from build123d import *

# Parameters (mm, degrees)
SKETCH1_R             = 22.5
SKETCH1_R_2           = 16.9
BOSS_EXTRUDE1_DEPTH   = 19
BOSS_EXTRUDE1_2_DEPTH = 19
BOSS_EXTRUDE2_DEPTH   = 9
CUT_EXTRUDE1_DEPTH    = 4
FILLET1_R             = 1
FILLET2_R             = 40
FILLET3_R             = 22.5
BOSS_EXTRUDE5_DEPTH   = 30
SKETCH6_R             = 27
CUT_EXTRUDE2_DEPTH    = 37
SKETCH7_R             = 4.5
CUT_EXTRUDE3_DEPTH    = 37


with BuildPart() as part:
    # Sketch1 → Boss-Extrude1 (new body, symmetric)
    with BuildSketch(Plane.XY):
        Circle(SKETCH1_R)
        Circle(SKETCH1_R_2, mode=Mode.SUBTRACT)
    extrude(amount=BOSS_EXTRUDE1_DEPTH, both=True)



with BuildPart() as body_2:
    # Sketch1 → Boss-Extrude1 2 (new body, symmetric)
    with BuildSketch(Plane.XY):
        with BuildLine():
            Line((-36, -201.2), (-27, -201.2))
            ThreePointArc((-27, -201.2), (0, -174.2), (27, -201.2))
            Line((27, -201.2), (36, -201.2))
            ThreePointArc((36, -201.2), (0, -165.2), (-36, -201.2))
        make_face()
    extrude(amount=BOSS_EXTRUDE1_2_DEPTH, both=True)


with BuildPart() as part_1:
    add(part.part)

    add(body_2.part)  # Boss-Extrude2 merges body 2
    # Sketch1<3> → Boss-Extrude2 (add, symmetric)
    with BuildSketch(Plane.XY):
        with BuildLine():
            ThreePointArc((10, -20.155644371), (0, -22.5), (-10, -20.155644371))
            Line((-10, -20.155644371), (-17.849697213, -169.936789841))
            ThreePointArc((-17.849697213, -169.936789841), (0, -165.2), (17.849697213, -169.936789841))
            Line((17.849697213, -169.936789841), (10, -20.155644371))
        make_face()
    extrude(amount=BOSS_EXTRUDE2_DEPTH, both=True)

    # Sketch2 → Cut-Extrude1 (cut)
    with BuildSketch(Plane.XY.offset(9)):
        with BuildLine():
            Line((-8, -145.6), (-8, -55.6))
            ThreePointArc((-8, -55.6), (0, -47.6), (8, -55.6))
            Line((8, -55.6), (8, -145.6))
            ThreePointArc((8, -145.6), (0, -153.6), (-8, -145.6))
        make_face()
    cut_extrude1 = extrude(amount=-CUT_EXTRUDE1_DEPTH, mode=Mode.SUBTRACT)

    # Mirror1: Cut-Extrude1 across plane
    add(cut_extrude1.mirror(Plane.XY), mode=Mode.SUBTRACT)

    # Fillet1
    fillet1_edges = [part_1.edges().sort_by_distance(p)[0] for p in [
        (8, -100.6, 5),
        (0, -153.6, 5),
        (-8, -100.6, 9),
        (0, -47.6, 5),
        (-8, -100.6, 5),
        (8, -100.6, 9),
        (0, -47.6, 9),
        (0, -153.6, 9),
        (8, -100.6, -9),
        (0, -47.6, -9),
        (-8, -100.6, -5),
        (0, -153.6, -9),
        (8, -100.6, -5),
        (0, -47.6, -5),
        (0, -153.6, -5),
        (-8, -100.6, -9),
    ]]
    fillet(fillet1_edges, radius=FILLET1_R)

    # Fillet2
    fillet2_edges = [part_1.edges().sort_by_distance(p)[0] for p in [
        (-17.849697213, -169.936789841, 0),
        (17.849697213, -169.936789841, 0),
    ]]
    fillet(fillet2_edges, radius=FILLET2_R)

    # Fillet3
    fillet3_edges = [part_1.edges().sort_by_distance(p)[0] for p in [
        (10, -20.155644371, 0),
        (-10, -20.155644371, 0),
    ]]
    fillet(fillet3_edges, radius=FILLET3_R)

    # Sketch3 → Boss-Extrude5 (add)
    with BuildSketch(Plane(origin=(0, -171.2, 0), x_dir=(-1, 0, 0), z_dir=(0, -1, 0))):
        with BuildLine():
            Line((38, -9), (-38, -9))
            ThreePointArc((-38, -9), (-47, 0), (-38, 9))
            Line((-38, 9), (38, 9))
            ThreePointArc((38, 9), (47, 0), (38, -9))
        make_face()
    extrude(amount=BOSS_EXTRUDE5_DEPTH)

    # Sketch6 → Cut-Extrude2 (cut)
    with BuildSketch(Plane(origin=(0, 0, -9), x_dir=(-1, 0, 0), z_dir=(0, 0, -1))):
        with Locations((0, -201.2)):
            Circle(SKETCH6_R)
    extrude(amount=-CUT_EXTRUDE2_DEPTH, mode=Mode.SUBTRACT)

    # Sketch7 → Cut-Extrude3 (cut)
    with BuildSketch(Plane(origin=(0, -171.2, 0), x_dir=(-1, 0, 0), z_dir=(0, -1, 0))):
        with Locations((-38, 0)):
            Circle(SKETCH7_R)
        with Locations((38, 0)):
            Circle(SKETCH7_R)
    extrude(amount=CUT_EXTRUDE3_DEPTH, mode=Mode.SUBTRACT)


solid = part_1.part
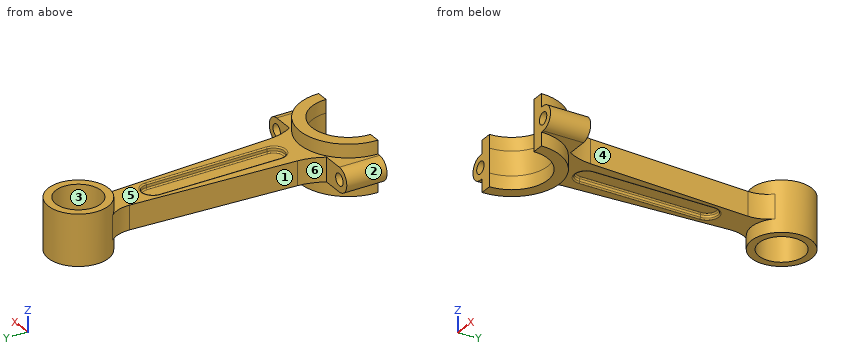
Read the model definition and answer for the solid it produces. Units are mm, in the model's axes. Face numbers are marked on the shaded views. A direction names the side the tool comes from. Give positions to 0.01 mm unless a question says otherwise; leave off trailing zeros. Write each loop counter-clockwise with the first axis right and the second up, starting at its lowest first coordinate (ties: lowest second). Pieces come first, ordered by that corner, then holes. Notation, with made-up numbers: (64, 11) - (76, 11) arc R21 ccw to (76, 48) - close; hole circle Ø4 at (20.25, 23.5). An arc over 180 degrees is marked (long way). Use CSV: the item, a comma, the result in double quotes. Start each with the question number.
(1) Find section C-C (y = 0). Give the vertices of the cut face in (x, z).
(2) Consider line 1 along Z through (x, y) = (38, -182.25); line 2 along Y through (x, z) = (7.5, -16); line 3 along X through (y, z) = (-183.5, 0). Determine where each line is inside the solid, lowest interval first.
(3) For the marked faces 1 and 2, determine the directions among +Z, -Z, +X, -X, +Y, -Y from which every point of the face is accessible in a straight line to the end or side of a thin tool.
(4) Determine the mould class of the marked faces 3, 4, 5 and 6 for opening direction X: +X half, -X half, draft (parallel to the pull), parting line (faces both ways), or undercut.
(5) Find section D-D (z = 15.5). Give the vertices of the cut face in (x, y), plus the area to 3 significant figures.
(6) Find section A-A (z = 0). Give the vertices of the cut face in (x, y).
(7) Given P1, Ø2, axis at y = -87.5, z = -6.5, coming from the +X side; P2, Ø9, axis at x = -40.5, z = 3, coming from the +Y side; P3, Ø3, axis at x = 1, z = 10, coming from the -Y side, each flat-ended and moving along its own axis, determine where each tip first touches the part or whether it passes through.
Findings below:
1,outline,"(-22.5, -19) - (-16.9, -19) - (-16.9, 19) - (-22.5, 19) - close; (16.9, -19) - (22.5, -19) - (22.5, 19) - (16.9, 19) - close"
2,line 1,"-9 to -4.5, 4.5 to 9"
2,line 2,"-175.26 to -165.99, -21.21 to -15.14, 15.14 to 21.21"
2,line 3,"-47 to -42.5, -33.5 to -20.39, 20.39 to 33.5, 42.5 to 47"
3,face 1,"+Z, -Z, -X"
3,face 2,"-X, +Y, -Y"
4,face 3,"undercut"
4,face 4,"+X half"
4,face 5,"draft"
4,face 6,"-X half"
5,outline,"(-36, -201.2) - (-27, -201.2) arc R27 cw to (27, -201.2) - (36, -201.2) arc R36 ccw to start; circle Ø45 at (0, 0); hole circle Ø33.8 at (0, 0)"
5,area,"1,580 mm2"
6,outline,"(-47, -201.2) - (-42.5, -201.2) - (-42.5, -171.2) - (-47, -171.2) - close; (-33.5, -201.2) - (-27, -201.2) arc R27 cw to (27, -201.2) - (33.5, -201.2) - (33.5, -171.2) - (22.48, -171.2) arc R40 cw to (16.96, -152.91) - (10.6, -31.69) arc R22.5 cw to (16.54, -15.26) arc R22.5 ccw (long way) to (-16.54, -15.26) arc R22.5 cw to (-10.6, -31.69) - (-16.96, -152.91) arc R40 cw to (-22.48, -171.2) - (-33.5, -171.2) - close; (42.5, -201.2) - (47, -201.2) - (47, -171.2) - (42.5, -171.2) - close; hole circle Ø33.8 at (0, 0)"
7,P1,"x = 13.58"
7,P2,"y = -171.2"
7,P3,"y = -174.32"
